from build123d import *

# Parameters (mm, degrees)
SKETCH2_W           = 50
SKETCH2_H           = 50
SKETCH2_R           = 8
SKETCH2_R_2         = 1.5
BOSS_EXTRUDE1_DEPTH = 5
SKETCH5_W           = 50
SKETCH5_H           = 5
BOSS_EXTRUDE2_DEPTH = 10
SKETCH6_R           = 1.5
CUT_EXTRUDE2_DEPTH  = 10
CHAMFER1_SIZE       = 1.5


with BuildPart() as part:
    # Sketch2 → Boss-Extrude1 (new body)
    with BuildSketch(Plane.XY):
        with Locations((0.61173319, 0.711954255)):
            Rectangle(SKETCH2_W, SKETCH2_H)
        with Locations((0.21173319, -6.688045745)):
            Circle(SKETCH2_R, mode=Mode.SUBTRACT)
        with Locations((-7.53826681, 13.735348013)):
            Circle(SKETCH2_R_2, mode=Mode.SUBTRACT)
        with Locations((7.96173319, 13.735348013)):
            Circle(SKETCH2_R_2, mode=Mode.SUBTRACT)
        with Locations((-15.28826681, 0.311954255)):
            Circle(SKETCH2_R_2, mode=Mode.SUBTRACT)
        with Locations((-7.53826681, -13.111439504)):
            Circle(SKETCH2_R_2, mode=Mode.SUBTRACT)
        with Locations((7.96173319, -13.111439504)):
            Circle(SKETCH2_R_2, mode=Mode.SUBTRACT)
        with Locations((15.71173319, 0.311954255)):
            Circle(SKETCH2_R_2, mode=Mode.SUBTRACT)
    extrude(amount=BOSS_EXTRUDE1_DEPTH)

    # Sketch5 → Boss-Extrude2 (add)
    with BuildSketch(Plane(origin=(0, 0, 0), x_dir=(-1, 0, 0), z_dir=(0, 0, -1))):
        with Locations((-0.61173319, -21.788045745)):
            Rectangle(SKETCH5_W, SKETCH5_H)
    extrude(amount=BOSS_EXTRUDE2_DEPTH)

    # Sketch6 → Cut-Extrude2 (cut)
    with BuildSketch(Plane.XZ.offset(24.288045745)):
        with Locations(Location((-19.38826681, -5, 0), (0, 0, 270))):
            Circle(SKETCH6_R)
        with Locations(Location((20.61173319, -5, 0), (0, 0, 270))):
            Circle(SKETCH6_R)
    extrude(amount=-CUT_EXTRUDE2_DEPTH, mode=Mode.SUBTRACT)

    # Chamfer1
    chamfer1_edges = [part.edges().sort_by_distance(p)[0] for p in [
        (-24.38826681, 0.711954255, 5),
        (25.61173319, 0.711954255, 5),
    ]]
    chamfer(chamfer1_edges, length=CHAMFER1_SIZE)


solid = part.part
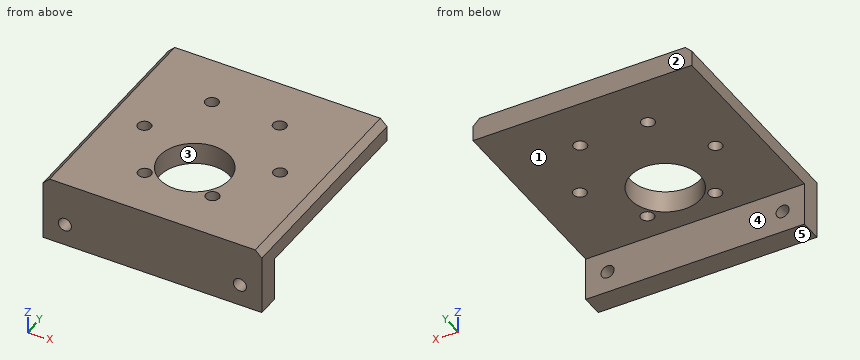
Read the model definition and answer for the solid it produces. Units are mm, in the model's axes. Face numbers are marked on the shaded views. A direction names the side the tool comes from. Give positions to 0.01 mm unless a question says otherwise; leave off trailing zeros. Loops run counter-clockwise (first coordinate to the right, second up) from the corner with the lowest first, then second, coordinate; pieces in that order, holes last. Notation, with made-up numbers: (82.5, 10.25) -> (139.5, 10.25) arc R32 cw to (139.5, 44.25) -> close; hole circle Ø8 at (-12, 13). An arc over 180 degrees is marked (long way). Use a Markdown table: item, result.
Q1. Section D-D, the plane z = -8.5 is taken. Determine the outline of the cut face in (x, y).
Solved:
| item | result |
|---|---|
| outline | (-24.39, -24.29) -> (25.61, -24.29) -> (25.61, -19.29) -> (-24.39, -19.29) -> close |
Q2. A tool of negligible diameter and unlimited length cuts with its end or side. For the marked faces 1 and 2, from which of +Z, -Z, +X, -X, +Y, -Y can it reach the whole face along a straight path? Write none if from no direction.
Solved:
| item | result |
|---|---|
| face 1 | -Z, +X, -X, +Y |
| face 2 | +Z, -Z, +X, -X, +Y |
Q3. Determine the mould class of the marked faces 3, 4 and 5 for opening direction Y: pulls with the +Y half, pulls with the -Y half, needs draft (parallel to the pull), parting line crosses it, or undercut.
Solved:
| item | result |
|---|---|
| face 3 | undercut |
| face 4 | pulls with the +Y half |
| face 5 | needs draft |
Q4. Section C-C, the plane y = 2.5 is taken. Determine the outline of the cut face in (x, z), then the cut area to 3 significant figures.
Solved:
| item | result |
|---|---|
| outline | (-24.39, 0) -> (25.61, 0) -> (25.61, 3.5) -> (24.11, 5) -> (-22.89, 5) -> (-24.39, 3.5) -> close |
| area | 248 mm^2 |
Q5. Each of these flat-tipped pins is pushed along its axis until it touches: pin 1 (5 mm diameter, centred on x = -7.54, y = 13.74, fed in from +Z); pin 2 (3.5 mm diameter, centred on x = 20.61, z = -5, fed in from +Y); pin 3 (2.5 mm diameter, centred on x = -15.29, y = 0.31, fed in from -Z); pin 4 (18.5 mm diameter, centred on x = 0.21, y = -6.69, fed in from -Z). Where does it stop, or does it pass through?
Solved:
| item | result |
|---|---|
| pin 1 | stops at z = 5 |
| pin 2 | stops at y = -19.29 |
| pin 3 | passes through |
| pin 4 | stops at z = 0 |
Q6. Section B-B, the plane x = -2.5 is taken. Determine the outline of the cut face in (y, z), then the cut area to 3 significant figures.
Solved:
| item | result |
|---|---|
| outline | (-24.29, -10) -> (-19.29, -10) -> (-19.29, 0) -> (-14.21, 0) -> (-14.21, 5) -> (-24.29, 5) -> close; (0.84, 0) -> (25.71, 0) -> (25.71, 5) -> (0.84, 5) -> close |
| area | 225 mm^2 |
Q7. Section A-A, the plane z = -5 is taken. Determine the outline of the cut face in (x, y).
Solved:
| item | result |
|---|---|
| outline | (-24.39, -24.29) -> (-20.89, -24.29) -> (-20.89, -19.29) -> (-24.39, -19.29) -> close; (-17.89, -24.29) -> (19.11, -24.29) -> (19.11, -19.29) -> (-17.89, -19.29) -> close; (22.11, -24.29) -> (25.61, -24.29) -> (25.61, -19.29) -> (22.11, -19.29) -> close |
Q8. Find the intervals of material crossed by line 1 along X through (y, z) = (-22.55, -5); line 2 along Y through (x, z) = (18.5, -3.5); line 3 along Z through (x, y) = (-19, -19), in increasing order.
Solved:
| item | result |
|---|---|
| line 1 | x = -24.39 to -20.89, -17.89 to 19.11, 22.11 to 25.61 |
| line 2 | y = -24.29 to -19.29 |
| line 3 | z = 0 to 5 |
